```python
from build123d import *

# Parameters (mm, degrees)
SKETCH1_W               = 178
SKETCH1_H               = 336
BOSS_EXTRUDE1_DEPTH     = 3
CUT_EXTRUDE1_DEPTH      = 348.600345224
CUT_EXTRUDE1_DEPTH_BACK = 348.600345224
SKETCH2_R               = 3.25


with BuildPart() as part:
    # Sketch1 → Boss-Extrude1 (new body)
    with BuildSketch(Plane.XY):
        with Locations((0, 168)):
            Rectangle(SKETCH1_W, SKETCH1_H)
    extrude(amount=BOSS_EXTRUDE1_DEPTH)

    # Sketch2 → Cut-Extrude1 (cut, two sides: drawn at the far end of the back side and taken through both)
    with BuildSketch(Plane.XY.offset(3).offset(-CUT_EXTRUDE1_DEPTH_BACK)):
        with Locations((-80, 250)):
            Circle(SKETCH2_R)
        with Locations((80, 250)):
            Circle(SKETCH2_R)
        with Locations((80, 30)):
            Circle(SKETCH2_R)
        with Locations((-80, 30)):
            Circle(SKETCH2_R)
    extrude(amount=CUT_EXTRUDE1_DEPTH + CUT_EXTRUDE1_DEPTH_BACK, mode=Mode.SUBTRACT)


solid = part.part
```
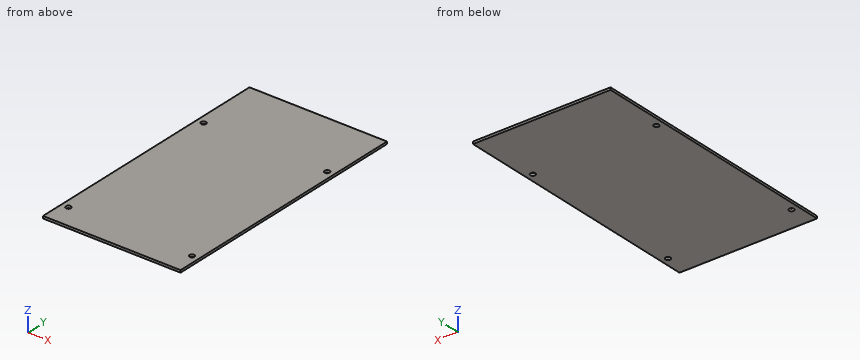
Can you work these out from the model? Positions are in its coordinate system, mm. Give positions to 0.01 mm unless a question says otherwise; leave off trailing zeros. Order: outer loops, then holes, each group sorted by start corner. A loop starts at its lowest first (then second) coordinate and runs counter-clockwise, first axis right, second up. Notation, with made-up numbers: M 34,51 L 47,51 A30 ccw 47,77 Z; hole C -36,-17 d8. An arc over 180 degrees is marked long. Write item = value, one per line. Start each with the question number.
Q1. Suppose I cut it at A-A (x = 80). Write out the boundary of the cut face in (y, z).
Q2. Suppose I cut it at B-B (y = 30). Write out the boundary of the cut face in (x, z), plus the area to 3 significant figures.
Q3. Will this pin go through, and if not, where does the flat tip stop? pin 1 Ø5 at (x, y) = (-80, 250) entering from +Z.
Q4. I need wall thicknesses on probe 1 along Y at (x, z) = (80, 1.55); probe 2 along X at (y, z) = (30, 1.9); probe 3 along X at (y, z) = (253, 1.05). Which ranges of each line are inside material? Lowest first, please. Write a range as [from, to].
Check result:
q1.outline = M 0,0 L 26.75,0 L 26.75,3 L 0,3 Z; M 33.25,0 L 246.75,0 L 246.75,3 L 33.25,3 Z; M 253.25,0 L 336,0 L 336,3 L 253.25,3 Z
q2.outline = M -89,0 L -83.25,0 L -83.25,3 L -89,3 Z; M -76.75,0 L 76.75,0 L 76.75,3 L -76.75,3 Z; M 83.25,0 L 89,0 L 89,3 L 83.25,3 Z
q2.area = 495 mm2
q3.pin_1 = through
q4.probe_1 = [0, 26.75], [33.25, 246.75], [253.25, 336]
q4.probe_2 = [-89, -83.25], [-76.75, 76.75], [83.25, 89]
q4.probe_3 = [-89, -81.25], [-78.75, 78.75], [81.25, 89]
